```python
from build123d import *

# Parameters (mm, degrees)
SKETCH1_R           = 2
BOSS_EXTRUDE1_DEPTH = 40
CUT_EXTRUDE1_DEPTH  = 82.663945533
CHAMFER1_SIZE       = 2.5
SKETCH3_W           = 12
SKETCH3_H           = 18
CUT_EXTRUDE2_DEPTH  = 82.663945533
FILLET1_R           = 4


with BuildPart() as part:
    # Sketch1 → Boss-Extrude1 (new body)
    with BuildSketch(Plane.XY):
        with BuildLine():
            Line((10, -9), (24.5, -9))
            Line((24.5, -9), (29.5, -14))
            Line((29.5, -14), (35.5, -14))
            Line((35.5, -14), (40.5, -9))
            Line((40.5, -9), (49.5, -9))
            Line((49.5, -9), (54.5, -14))
            Line((54.5, -14), (60.5, -14))
            Line((60.5, -14), (65.5, -9))
            Line((65.5, -9), (70, -9))
            Line((70, -9), (70, -1))
            Line((70, -1), (10, -1))
            Line((10, -1), (1.949288889, 3.492888894))
            ThreePointArc((1.949288889, 3.492888894), (-3.566315144, 1.811462473), (-1.670874988, -3.634305542))
            Line((-1.670874988, -3.634305542), (10, -9))
        make_face()
        Circle(SKETCH1_R, mode=Mode.SUBTRACT)
    extrude(amount=BOSS_EXTRUDE1_DEPTH)

    # Sketch2 → Cut-Extrude1 (cut, through all)
    with BuildSketch(Plane.XZ.offset(9)):
        with BuildLine():
            Line((47.25, 31), (47.25, 9))
            ThreePointArc((47.25, 9), (45, 6.75), (42.75, 9))
            Line((42.75, 9), (42.75, 31))
            ThreePointArc((42.75, 31), (45, 33.25), (47.25, 31))
        make_face()
    extrude(amount=-CUT_EXTRUDE1_DEPTH, mode=Mode.SUBTRACT)

    # Chamfer1
    chamfer1_edges = [part.edges().sort_by_distance(p)[0] for p in [
        (42.75, -1, 20),
        (45, -1, 6.75),
        (47.25, -1, 20),
        (45, -1, 33.25),
    ]]
    chamfer(chamfer1_edges, length=CHAMFER1_SIZE)

    # Sketch3 → Cut-Extrude2 (cut, through all)
    with BuildSketch(Plane.XZ.offset(9)):
        with Locations((2, 20)):
            Rectangle(SKETCH3_W, SKETCH3_H)
    extrude(amount=-CUT_EXTRUDE2_DEPTH, mode=Mode.SUBTRACT)

    # Fillet1
    # the kernel refuses this fillet: 4 mm, written as the material it takes off along each edge
    with BuildSketch(Plane(origin=(8, 0.116147091, 29), x_dir=(0.8732222234943452, -0.4873222223494347, 0), z_dir=(0, 0, -1))) as fillet1_piece_1:
        with BuildLine():
            CenterArc((5.724945872, 2.05028607), FILLET1_R, 150.835269547, 60)
            Line((2.232056978, 3.999574959), (0, 0))
            Line((0, 0), (2.290367728, 0))
        make_face()
    extrude(amount=18, mode=Mode.SUBTRACT)
    with BuildSketch(Plane(origin=(8, -8.080498341, 11), x_dir=(0.9085763855616094, -0.4177187470054484, 0), z_dir=(0, 0, 1))) as fillet1_piece_2:
        with BuildLine():
            CenterArc((FILLET1_R * 0.640872096444, FILLET1_R), FILLET1_R, 204.690646006, 65.309353994)
            Line((-FILLET1_R * 0.267704289117, FILLET1_R * 0.582281252995), (0, 0))
            Line((0, 0), (FILLET1_R * 0.640872096444, 0))
        make_face()
    extrude(amount=18, mode=Mode.SUBTRACT)


solid = part.part
```
Verification items for the finished model (mm, model axes). A direction names the side the tool comes from. Give positions to 0.01 mm unless a question says otherwise; leave off trailing zeros. Loops run counter-clockwise (first coordinate to the right, second up) from the corner with the lowest first, then second, coordinate; pieces in that order, holes last. Notation, with made-up numbers: M 9,77.5 L 41,77.5 A30 cw 41,106.5 Z; hole C 66.25,40 d4. An arc over 180 degrees is marked long. Return JSON: item names as keys, results as strings.
1) Section check C-C, the plane x = 59.5. Enter the section's corners in (y, z).
Findings:
{"outline": "M -14,0 L -1,0 L -1,40 L -14,40 Z"}
2) Material ranges on L1, parallel to Z at x = 45, y = -8.25; L2, parallel to Z at x = 6, y = 1; L3, parallel to Y at x = 24, z = 38.5, recorded low to high. Write a range as [from, to].
Findings:
{"L1": "z = [0, 6.75], [33.25, 40]", "L2": "z = [0, 11], [29, 40]", "L3": "y = [-9, -1]"}
3) Mould release check, pull along X, two halves, no side actions. Record for faces 1 (the flat face through (6.031, 1.215, 5.423)), 2 (the flat face through (34, -1, 20)), 3 (the flat face through (38, -11.5, 19.7)): released by +X, released by -X, zero draft, split by the parting line, or undercut.
Findings:
{"face 1": "released by +X", "face 2": "zero draft", "face 3": "undercut"}
4) Section check B-B, the plane z = 23. Enter the section's corners in (x, y), and give its area (3 significant figures).
Findings:
{"outline": "M 8,-5.52 A4 ccw 10.03,-9 L 24.5,-9 L 29.5,-14 L 35.5,-14 L 40.5,-9 L 42.75,-9 L 42.75,-3.5 L 40.25,-1 L 10,-1 A4 ccw 8,-4.46 Z; M 47.25,-9 L 49.5,-9 L 54.5,-14 L 60.5,-14 L 65.5,-9 L 70,-9 L 70,-1 L 49.75,-1 L 47.25,-3.5 Z", "area": "560 mm2"}
5) Tool access check on faces 4 (the flat face through (41.52, -2.27, 19.85)), 5 (the flat face through (68, -9, 20)), 6 (the cylindrical face through (8.53, -7.51, 19.87)), 7 (the flat face through (42, -9, 20)). Record the directions out of +Z, -Z, +X, -X, +Y, -Y that give a thin tool (end or side, any length) a straight path to the whole face; none if there is none.
Findings:
{"face 4": "+Y", "face 5": "+Z, -Z, +X, -Y", "face 6": "-X, -Y", "face 7": "+Z, -Z, -Y"}
6) Section check A-A, the plane z = 37. Enter the section's corners in (x, y).
Findings:
{"outline": "M -1.67,-3.63 L 10,-9 L 24.5,-9 L 29.5,-14 L 35.5,-14 L 40.5,-9 L 49.5,-9 L 54.5,-14 L 60.5,-14 L 65.5,-9 L 70,-9 L 70,-1 L 10,-1 L 1.95,3.49 A4 ccw long Z; hole C 0,0 d4"}
7) Section check D-D, the plane x = 11. Enter the section's corners in (y, z).
Findings:
{"outline": "M -9,0 L -1,0 L -1,40 L -9,40 Z"}
8) Gauge pin test, flat ends, axial feed: P1, Ø4.5, axis at x = 14, z = 21.5, coming from the -Y side; P2, Ø1.6, axis at y = -6, z = 22, coming from the -X side; P3, Ø6, axis at x = 50.5, z = 23.5, coming from the +Y side. Record the tip position at first contact, or that the pin passes through.
Findings:
{"P1": "stops at y = -9", "P2": "stops at x = 8", "P3": "stops at y = -1"}
